The listing builds one solid part. Answer for the finished solid, in the listing's coordinates (mm). Coordinates: 2 decimals unless noted, no trailing zeros. Use one line per item in the form item = value. Start each with the question number.
Item 1: Section A-A, the plane z = 3.3 is taken. Count the separate pieces of the cut face and the enclosed holes in it, and give its area (3 significant figures).
Item 2: This flat-tipped pin is pushed along its axis until it touches: pin 1 Ø0.7 at (x, z) = (118.5, 3) entering from +Y. Where does it stop, or does it pass through?
Item 3: Consider line 1 along Y through (x, z) = (50, 1.5) (3 decimals); line 2 along Y through (x, z) = (39.5, 3.7); line 3 along Y through (x, z) = (112, 3.8). Determine where each line is inside the solid, lowest interval first. Write a range as [from, to].
from build123d import *

# Parameters (mm, degrees)
SKETCH_1_W             = 218.58974427
SKETCH_1_H             = 22.5
EXTRUDE_1_DEPTH        = 6
EXTRUDE_2_DEPTH        = 6
PATTERN_LINEAR_1_COUNT = 35
PATTERN_LINEAR_1_PITCH = 6.283185307
SKETCH_3_R             = 1.525
CUT_EXTRUDE_1_DEPTH    = 10
PATTERN_LINEAR_2_COUNT = 7
PATTERN_LINEAR_2_PITCH = 30
FILLET_1_R             = 3
SKETCH_4_R             = 4.5
CUT_EXTRUDE_2_DEPTH    = 10


with BuildPart() as part:
    # 草图1 → 拉伸1 (new body)
    with BuildSketch(Plane.XY):
        with Locations((109.294872135, -11.25)):
            Rectangle(SKETCH_1_W, SKETCH_1_H)
    extrude(amount=EXTRUDE_1_DEPTH)

    # 草图2 → 拉伸2 (add)
    with BuildSketch(Plane.XY.offset(6)):
        Polygon((0, 0), (1.637866054, 4.5), (3.323577771, 4.5), (4.961443825, 0), align=None)
    extrude_2 = extrude(amount=-EXTRUDE_2_DEPTH)

    # 阵列(线性)1: 拉伸2 ×35
    with Locations(*[(i * PATTERN_LINEAR_1_PITCH, 0, 0) for i in range(1, PATTERN_LINEAR_1_COUNT)]):
        add(extrude_2)

    # 草图3 → 切除-拉伸1 (cut)
    with BuildSketch(Plane.XY.offset(6)):
        with Locations((20, -12.5)):
            Circle(SKETCH_3_R)
    cut_extrude_1 = extrude(amount=-CUT_EXTRUDE_1_DEPTH, mode=Mode.SUBTRACT)

    # 阵列(线性)2: 切除-拉伸1 ×7
    with Locations(*[(i * PATTERN_LINEAR_2_PITCH, 0, 0) for i in range(1, PATTERN_LINEAR_2_COUNT)]):
        add(cut_extrude_1, mode=Mode.SUBTRACT)

    # 圆角1
    fillet_1_edges = [part.edges().sort_by_distance(p)[0] for p in [
        (218.58974427, -22.5, 3),
        (0, -22.5, 3),
    ]]
    fillet(fillet_1_edges, radius=FILLET_1_R)

    # 草图4 → 切除-拉伸2 (cut)
    with BuildSketch(Plane.XY.offset(6)):
        with Locations((9, -12.5)):
            Circle(SKETCH_4_R)
        with Locations((211, -12.5)):
            Circle(SKETCH_4_R)
        with BuildLine():
            Line((29, -7.5), (41, -7.5))
            ThreePointArc((41, -7.5), (46, -12.5), (41, -17.5))
            Line((41, -17.5), (29, -17.5))
            ThreePointArc((29, -17.5), (24, -12.5), (29, -7.5))
        make_face()
        with BuildLine():
            Line((71, -7.5), (59, -7.5))
            ThreePointArc((59, -7.5), (54, -12.5), (59, -17.5))
            Line((59, -17.5), (71, -17.5))
            ThreePointArc((71, -17.5), (76, -12.5), (71, -7.5))
        make_face()
        with BuildLine():
            Line((89, -7.5), (101, -7.5))
            ThreePointArc((101, -7.5), (106, -12.5), (101, -17.5))
            Line((101, -17.5), (89, -17.5))
            ThreePointArc((89, -17.5), (84, -12.5), (89, -7.5))
        make_face()
        with BuildLine():
            Line((191, -7.5), (179, -7.5))
            ThreePointArc((179, -7.5), (174, -12.5), (179, -17.5))
            Line((179, -17.5), (191, -17.5))
            ThreePointArc((191, -17.5), (196, -12.5), (191, -7.5))
        make_face()
        with BuildLine():
            Line((149, -7.5), (161, -7.5))
            ThreePointArc((161, -7.5), (166, -12.5), (161, -17.5))
            Line((161, -17.5), (149, -17.5))
            ThreePointArc((149, -17.5), (144, -12.5), (149, -7.5))
        make_face()
        with BuildLine():
            Line((131, -7.5), (119, -7.5))
            ThreePointArc((119, -7.5), (114, -12.5), (119, -17.5))
            Line((119, -17.5), (131, -17.5))
            ThreePointArc((131, -17.5), (136, -12.5), (131, -7.5))
        make_face()
    extrude(amount=-CUT_EXTRUDE_2_DEPTH, mode=Mode.SUBTRACT)


solid = part.part
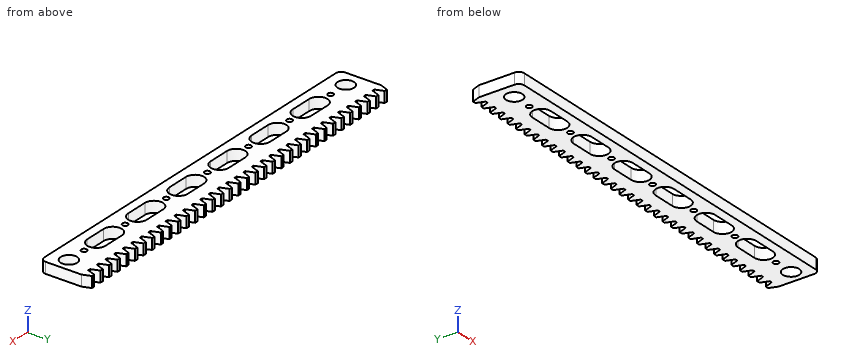
Response:
q1.separate_pieces = 1
q1.enclosed_holes = 15
q1.area = 4,070 mm2
q2.pin_1 = 0
q3.line_1 = [-22.5, -14.025], [-10.975, 0]
q3.line_2 = [-22.5, -17.5], [-7.5, 4.5]
q3.line_3 = [-22.5, 0]
